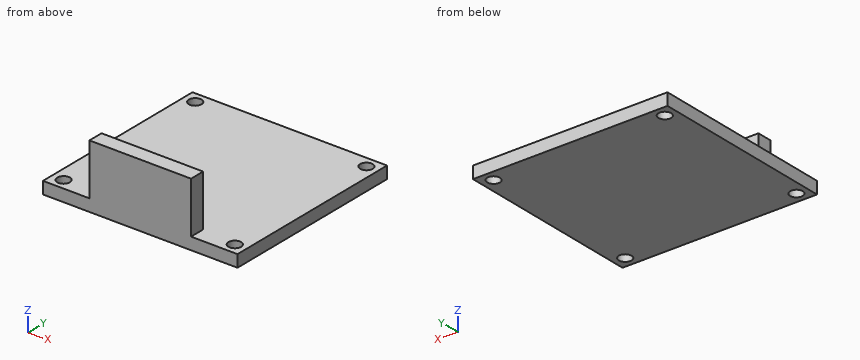
```python
from build123d import *

# Parameters (mm, degrees)
F0_W     = 32.16
F0_H     = 31
F1_DEPTH = 2
F3_D     = 2.1
F3_DEPTH = 5
F4_W     = 16.8
F4_H     = 2.5
F5_DEPTH = 8.5


with BuildPart() as f1:
    # F0 (on Top) → F1 (new body)
    with BuildSketch(Plane.XY):
        Rectangle(F0_W, F0_H)
    extrude(amount=F1_DEPTH)

    # F3
    with Locations(Plane.XY.offset(2)):
        with Locations((-14.155587, 13.645), (14.155587, 13.645), (-14.155587, -13.645), (14.155587, -13.645)):
            Hole(F3_D / 2, depth=F3_DEPTH)

    # F4 (on face) → F5 (join)
    with BuildSketch(Plane.XY.offset(2)):
        with Locations((0, -14.25)):
            Rectangle(F4_W, F4_H)
    extrude(amount=F5_DEPTH)


solid = f1.part
```
Source: CAD feature listing. Evaluate the final solid. Frame: model axes, mm. Give positions to 0.01 mm unless a question says otherwise; leave off trailing zeros. Write each loop counter-clockwise with the first axis right and the second up, starting at its lowest first coordinate (ties: lowest second). Pieces come first, ordered by that corner, then holes.
1. Section query A-A (x = 14.5). Return the cut outline in (y, z).
2. Section query D-D (y = 5.5). Return the cut outline in (x, z), then the cut area to 3 significant figures.
3. Material intervals for line 1 along Y through (x, z) = (-7, 4.25); line 2 along Z through (x, y) = (-3, -9.5), sorted ascending.
4. Section query B-B (x = 6). Return the cut outline in (y, z).
5. First-contact query: pin 1 (1.2 mm diameter, centred on y = -14, z = 8, fed in from -X); pin 2 (1.3 mm diameter, centred on x = 14.16, y = -13.64, fed in from +Z); pin 3 (2.5 mm diameter, centred on x = -14.16, y = 13.64, fed in from +Z); pin 4 (0.8 mm diameter, centred on y = -14, z = 4.5, fed in from +X). Flat tips, straight axial feed; report the tip coordinate or a pass-through.
6. Section query C-C (z = 4). Return the cut outline in (x, y), then the cut area to 3 significant figures.
Output values:
1. outline: (-15.5, 0) - (-14.64, 0) - (-14.64, 2) - (-15.5, 2) - close; (-12.65, 0) - (12.65, 0) - (12.65, 2) - (-12.65, 2) - close; (14.64, 0) - (15.5, 0) - (15.5, 2) - (14.64, 2) - close
2. outline: (-16.08, 0) - (16.08, 0) - (16.08, 2) - (-16.08, 2) - close
2. area: 64.3 mm2
3. line 1: y = -15.5 to -13
3. line 2: z = 0 to 2
4. outline: (-15.5, 0) - (15.5, 0) - (15.5, 2) - (-13, 2) - (-13, 10.5) - (-15.5, 10.5) - close
5. pin 1: stops at x = -8.4
5. pin 2: passes through
5. pin 3: stops at z = 2
5. pin 4: stops at x = 8.4
6. outline: (-8.4, -15.5) - (8.4, -15.5) - (8.4, -13) - (-8.4, -13) - close
6. area: 42.0 mm2
